from build123d import *

# Parameters (mm, degrees)
F0_W     = 90.2919955552
F0_H     = 55.083796382
F1_DEPTH = 12.7
F2_T     = -2.54
F3_R     = 8.3062100312
F4_DEPTH = 25.4


with BuildPart() as f1:
    # F0 (on Front) → F1 (new body, symmetric)
    with BuildSketch(Plane.XZ):
        with Locations((4.5429933816, -1.2777205557)):
            Rectangle(F0_W, F0_H)
    extrude(amount=F1_DEPTH, both=True)

    # F2
    f2_openings = [f1.faces().sort_by_distance(p)[0] for p in [
        (4.542993, -12.7, -1.277721),
    ]]
    offset(amount=F2_T, openings=f2_openings)

    # F3 (on face) → F4 (cut)
    with BuildSketch(Plane(origin=(0, 0, -28.8196187466), x_dir=(1, 0, 0), z_dir=(0, 0, -1))):
        with Locations((-27.4217892438, 0)):
            Circle(F3_R)
    extrude(amount=-F4_DEPTH, mode=Mode.SUBTRACT)


solid = f1.part
Here's how the part is built. I have some questions about the finished solid (model axes, mm). A direction names the side the tool comes from. Round coordinates to 2 decimals unless told otherwise and drop trailing zeros. Write each loop counter-clockwise with the first axis right and the second up, starting at its lowest first coordinate (ties: lowest second). Pieces come first, ordered by that corner, then holes.
1. If we mould it in two halves opening along Z, with no side actions, what happens to faces 1 (the flat face through (4, 0, -28.82)), 2 (the flat face through (47.149, -1, -2)), 3 (the cylindrical face through (-35.72, -0.37, -27.57))? For each: released by +Z, released by -Z, zero draft, split by the parting line, or undercut.
2. Suppose I cut it at B-B (x = 23). List the corners of the cut face in (y, z) for me, and give its area (3 significant figures).
3. Suppose I cut it at C-C (z = 15.5). List the corners of the cut face in (x, y) for me, and give its area (3 significant figures).
4. Suppose I cut it at A-A (y = -9.75). List the corners of the cut face in (x, z) for me, and give its area (3 significant figures).
5. Suppose I cut it at D-D (y = 0). List the corners of the cut face in (x, z) for me, and give its area (3 significant figures).
6. For faces 4 (the flat face through (4, 10.16, -1)), 5 (the flat face through (4, 0, 26.264)), which set-ups out of +Z, -Z, +X, -X, +Y, -Y let a thin tool reach every point of the face, with its end or its side?
7. I need wall thicknesses on L1, parallel to X at y = -5, z = -6; L2, parallel to Z at x = 1, y = 2.5; L3, parallel to X at y = 0, z = -27. Which ranges of each line are inside material? Lowest first, please.
8. Will this pin go through, and if not, where does the flat tip stop? pin 1 Ø8 at (x, z) = (-4, 8) entering from -Y.
Answer sheet:
1. face 1: released by -Z
1. face 2: undercut
1. face 3: zero draft
2. outline: (-12.7, -28.82) - (12.7, -28.82) - (12.7, 26.26) - (-12.7, 26.26) - (-12.7, 23.72) - (10.16, 23.72) - (10.16, -26.28) - (-12.7, -26.28) - close
2. area: 256 mm2
3. outline: (-40.6, -12.7) - (-38.06, -12.7) - (-38.06, 10.16) - (47.15, 10.16) - (47.15, -12.7) - (49.69, -12.7) - (49.69, 12.7) - (-40.6, 12.7) - close
3. area: 345 mm2
4. outline: (-40.6, -28.82) - (49.69, -28.82) - (49.69, 26.26) - (-40.6, 26.26) - close; hole (-38.06, -26.28) - (47.15, -26.28) - (47.15, 23.72) - (-38.06, 23.72) - close
4. area: 713 mm2
5. outline: (-40.6, -28.82) - (-35.73, -28.82) - (-35.73, -26.28) - (-38.06, -26.28) - (-38.06, 23.72) - (47.15, 23.72) - (47.15, -26.28) - (-19.12, -26.28) - (-19.12, -28.82) - (49.69, -28.82) - (49.69, 26.26) - (-40.6, 26.26) - close
5. area: 671 mm2
6. face 4: -Y
6. face 5: +Z, +X, -X, +Y, -Y
7. L1: x = -40.6 to -38.06, 47.15 to 49.69
7. L2: z = -28.82 to -26.28, 23.72 to 26.26
7. L3: x = -40.6 to -35.73, -19.12 to 49.69
8. pin 1: stops at y = 10.16
